Source: CAD feature listing. Evaluate the final solid. Frame: model axes, mm. A direction names the side the tool comes from. Round coordinates to 2 decimals unless told otherwise and drop trailing zeros. Write each loop counter-clockwise with the first axis right and the second up, starting at its lowest first coordinate (ties: lowest second). Pieces come first, ordered by that corner, then holes. Notation, with made-up numbers: (-3, -29.75) - (12, -29.75) arc R23 cw to (12, -5.75) - close; hole circle Ø9 at (24, -35). An arc over 180 degrees is marked (long way). Write item = value, one per line. Start each with the question number.
```python
from build123d import *

# Parameters (mm, degrees)
F0_W      = 96.52
F0_H      = 2.54
F1_DEPTH  = 142.24
F2_W      = 10
F2_H      = 142.24
F3_DEPTH  = 0.9017
F5_DEPTH  = 142.241
F8_DEPTH  = 5
F9_SIZE   = 4.99999
F10_W     = 9.9
F10_H     = 142.24
F11_DEPTH = 3.4427


# Not quite as in the source:
# - a fillet or chamfer is up to 0.001 mm smaller than in the source, because OpenCascade refuses the exact size


with BuildPart() as f1:
    # F0 (on Front) → F1 (new body)
    with BuildSketch(Plane.XZ):
        with Locations((-48.26, 1.27)):
            Rectangle(F0_W, F0_H)
    extrude(amount=F1_DEPTH)

    # F2 (on face) → F3 (join)
    with BuildSketch(Plane(origin=(0, 0, 0), x_dir=(1, 0, 0), z_dir=(0, 0, -1))):
        with Locations((-81.614, 71.12)):
            Rectangle(F2_W, F2_H)
        with Locations((-9.0132, 71.12)):
            Rectangle(F2_W, F2_H)
    extrude(amount=F3_DEPTH)

    # F4 (on face) → F5 (cut, through all)
    with BuildSketch(Plane.XZ.offset(142.24)):
        Polygon((-86.614, 0), (-86.614, -0.9017), (-86.0057956704, 0), align=None)
        Polygon((-77.2222043296, 0), (-76.614, -0.9017), (-76.614, 0), align=None)
        Polygon((-14.0132, 0), (-14.0132, -0.9017), (-13.4049956704, 0), align=None)
        Polygon((-4.6214043296, 0), (-4.0132, -0.9017), (-4.0132, 0), align=None)
    extrude(amount=-F5_DEPTH, mode=Mode.SUBTRACT)

    # F7 (on face) → F8 (join)
    with BuildSketch(Plane.XY.offset(2.54)):
        Polygon((-15.67, -5), (-85.52, -5), (-85.52, -105.076), (-80.52, -105.076), (-80.52, -10), (-15.67, -10), align=None)
    extrude(amount=F8_DEPTH)

    # F9 (size 5 in the source; OpenCascade refuses exactly that, so slightly less here)
    f9_edges = [f1.edges().sort_by_distance(p)[0] for p in [
        (-85.52, -55.038, 7.54),
        (-50.595, -5, 7.54),
    ]]
    chamfer(f9_edges, length=F9_SIZE)

    # F10 (on face) → F11 (cut, through all)
    with BuildSketch(Plane.XY.offset(2.54)):
        with Locations((-91.57, -71.12)):
            Rectangle(F10_W, F10_H)
    extrude(amount=-F11_DEPTH, mode=Mode.SUBTRACT)


solid = f1.part
```
(1) Reachability of faces 1 (the flat face through (-15.67, -8, 4)), 2 (the flat face through (-82, -105.076, 4)), 3 (the flat face through (-82.985, -54.337, 5.075)), 4 (the flat face through (-82, -72, -0.902)), 5 (the flat face through (-49, -10, 5)) from +Z, -Z, +X, -X, +Y, -Y: full face, straight path, thin tool, end or side. Return the list, or none.
(2) Contact query for flat-ended pins moving along their axis: P1, Ø4, axis at x = -82.5, z = 5, coming from the -Y side; P2, Ø1.5, axis at y = -47, z = 6.5, coming from the -X side; P3, Ø8, axis at x = -50, y = -71.5, coming from the -Z side; P4, Ø3, axis at y = -69, z = 3, coming from the -X side. Output: stop coordinate, or through.
(3) Pull-direction query (X, two-part tool) for faces 6 (the flat face through (-45, -72, 0)), 7 (the flat face through (0, -70, 1)), 8 (the flat face through (-44, -142.24, 1)); classes: +X half, -X half, draft (parallel to the pull), parting line (faces both ways), or undercut.
(4) Section D-D (y = -129). Return the cut outline in (x, z) (3 decimals).
(5) Section C-C (z = 5.75). Return the cut outline in (x, y).
(6) Ray query, L1, parallel to Z at x = -45, y = -108; L2, parallel to Z at x = -5.5, y = -74; L3, parallel to X at y = -114.5, z = -0.5. Return the intervals inside material, ascending. Write a range as from..to.
Solution:
q1.face_1 = +Z, +X, +Y, -Y
q1.face_2 = +Z, +X, -X, -Y
q1.face_3 = +Z, -X, +Y, -Y
q1.face_4 = -Z, +X, -X, +Y, -Y
q1.face_5 = +Z, +X, -Y
q2.P1 = -105.08
q2.P2 = -82.31
q2.P3 = 0
q2.P4 = -86.62
q3.face_6 = undercut
q3.face_7 = +X half
q3.face_8 = draft
q4.outline = (-86.62, 0) - (-86.006, 0) - (-86.614, -0.902) - (-76.614, -0.902) - (-77.222, 0) - (-13.405, 0) - (-14.013, -0.902) - (-4.013, -0.902) - (-4.621, 0) - (0, 0) - (0, 2.54) - (-86.62, 2.54) - close
q5.outline = (-82.31, -105.08) - (-80.52, -105.08) - (-80.52, -10) - (-15.67, -10) - (-15.67, -8.21) - (-82.31, -8.21) - close
q6.L1 = 0..2.54
q6.L2 = -0.9..2.54
q6.L3 = -86.34..-76.88, -13.74..-4.28
